Input: part model. Units: mm. Frame: model coordinates. Give positions to 0.01 mm unless a question says otherwise; leave off trailing zeros. Order: outer loops, then holes, each group sorted by start corner. A loop starts at its lowest first (then second) coordinate and runs counter-clockwise, first axis right, second up. Notation, with made-up numbers: (-26.5, 2) - (13.5, 2) arc R26 cw to (13.5, 21) - close; hole circle Ø1 at (19, 68). An arc over 180 degrees is marked (long way). Answer in a Markdown table with one row per item. Add a question column.
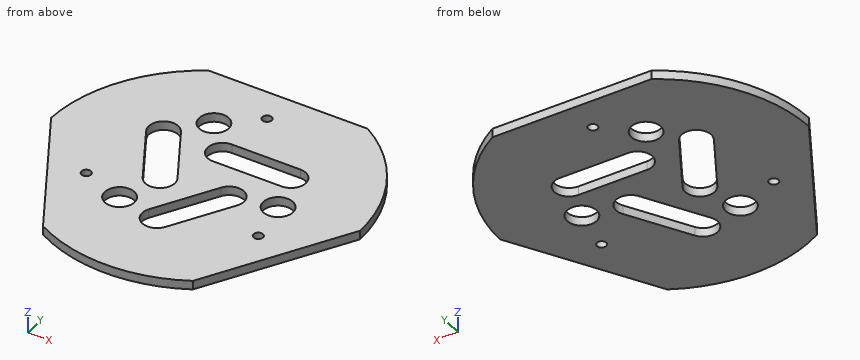
from build123d import *

# Parameters (mm, degrees)
SKETCH_1_R               = 1.6
SKETCH_1_R_2             = 5
EXTRUDE_1_DEPTH          = 1.5
CUT_EXTRUDE_1_DEPTH      = 75.301116494
PATTERN_CIRCULAR_1_COUNT = 3
SKETCH_3_R               = 5
CUT_EXTRUDE_3_DEPTH      = 75.301116494
PATTERN_CIRCULAR_3_COUNT = 3


with BuildPart() as part:
    # 草图1 → 凸台-拉伸1 (new, symmetric)
    with BuildSketch(Plane.XY):
        with BuildLine():
            Line((25.450325887, -45.918742494), (52.491960453, 0.918742494))
            ThreePointArc((52.491960453, 0.918742494), (45.466333699, 26.25), (27.041634566, 45))
            Line((27.041634566, 45), (-27.041634566, 45))
            ThreePointArc((-27.041634566, 45), (-45.466333699, 26.25), (-52.491960453, 0.918742494))
            Line((-52.491960453, 0.918742494), (-25.450325887, -45.918742494))
            ThreePointArc((-25.450325887, -45.918742494), (0, -52.5), (25.450325887, -45.918742494))
        make_face()
        with Locations((0, 33.75)):
            Circle(SKETCH_1_R, mode=Mode.SUBTRACT)
        with Locations((29.228357378, -16.875)):
            Circle(SKETCH_1_R, mode=Mode.SUBTRACT)
        with Locations((-29.228357378, -16.875)):
            Circle(SKETCH_1_R, mode=Mode.SUBTRACT)
        with Locations((0, -25)):
            Circle(SKETCH_1_R_2, mode=Mode.SUBTRACT)
        with Locations((-21.650635095, 12.5)):
            Circle(SKETCH_1_R_2, mode=Mode.SUBTRACT)
        with Locations((21.650635095, 12.5)):
            Circle(SKETCH_1_R_2, mode=Mode.SUBTRACT)
    extrude(amount=EXTRUDE_1_DEPTH, both=True)

    # 草图2 → 切除-拉伸1 (cut, through all)
    with BuildSketch(Plane.XY.offset(1.5)):
        with BuildLine():
            Line((-17.320508076, 15), (-5.669872981, -5.179491924))
            ThreePointArc((-5.669872981, -5.179491924), (-7.5, -12.009618943), (-14.330127019, -10.179491924))
            Line((-14.330127019, -10.179491924), (-25.980762114, 10))
            ThreePointArc((-25.980762114, 10), (-24.150635095, 16.830127019), (-17.320508076, 15))
        make_face()
    cut_extrude_1 = extrude(amount=-CUT_EXTRUDE_1_DEPTH, mode=Mode.SUBTRACT)

    # 阵列(圆周)1: 切除-拉伸1 ×3 about axis
    pattern_circular_1_axis = Axis((0, 0, 0), (0, 0, 1))
    for i in range(1, PATTERN_CIRCULAR_1_COUNT):
        add(cut_extrude_1.rotate(pattern_circular_1_axis, i * 360 / PATTERN_CIRCULAR_1_COUNT), mode=Mode.SUBTRACT)

    # 草图3 → 切除-拉伸3 (cut, through all)
    with BuildSketch(Plane.XY.offset(1.5)):
        with Locations((-11.650635095, 23.680339887)):
            Circle(SKETCH_3_R)
    cut_extrude_3 = extrude(amount=-CUT_EXTRUDE_3_DEPTH, mode=Mode.SUBTRACT)

    # 阵列(圆周)3: 切除-拉伸3 ×3 about axis
    pattern_circular_3_axis = Axis((0, 0, 0), (0, 0, 1))
    for i in range(1, PATTERN_CIRCULAR_3_COUNT):
        add(cut_extrude_3.rotate(pattern_circular_3_axis, i * 360 / PATTERN_CIRCULAR_3_COUNT), mode=Mode.SUBTRACT)


solid = part.part
Q1. Section C-C, the plane y = -25. Return loops of the section in (x, z), then the cut area to 3 significant figures.
Q2. Section A-A, the plane x = 0. Return loops of the section in (y, z).
Q3. Section B-B, the plane z = 0.9. State how many separate pieces and enclosed holes the cut face has, then the cut area to 3 significant figures.
Q4. Line query: probe 1 along X at (y, z) = (-10.5, -0.7); probe 2 along X at (y, z) = (-23.5, 1.2); probe 3 along Y at (x, z) = (23.5, 1.2). Output: solid intervals per line, ascending.
Q5. Section D-D, the plane y = 22.5. Return loops of the section in (x, z), then the cut area to 3 significant figures.
Q6. Contact query for flat-ended pins moving along their axis: P1, Ø16, axis at x = -11.65, y = 23.68, coming from the -Z side; P2, Ø1.5, axis at x = 10, z = 0, coming from the -Y side. Output: stop coordinate, or through.
Computed:
| question | item | result |
|---|---|---|
| 1 | outline | (-37.53, -1.5) - (-18.63, -1.5) - (-18.63, 1.5) - (-37.53, 1.5) - close; (-10.74, -1.5) - (-5, -1.5) - (-5, 1.5) - (-10.74, 1.5) - close; (5.77, -1.5) - (37.53, -1.5) - (37.53, 1.5) - (5.77, 1.5) - close |
| 1 | area | 169 mm^2 |
| 2 | outline | (-52.5, -1.5) - (-30, -1.5) - (-30, 1.5) - (-52.5, 1.5) - close; (-15, -1.5) - (7.5, -1.5) - (7.5, 1.5) - (-15, 1.5) - close; (17.5, -1.5) - (32.15, -1.5) - (32.15, 1.5) - (17.5, 1.5) - close; (35.35, -1.5) - (45, -1.5) - (45, 1.5) - (35.35, 1.5) - close |
| 3 | separate pieces | 1 |
| 3 | enclosed holes | 9 |
| 3 | area | 6,640 mm^2 |
| 4 | probe 1 | x = -45.9 to -14.13, -5.87 to 2.6, 14.15 to 45.9 |
| 4 | probe 2 | x = -38.39 to -19.43, -9.94 to -4.77, 6.64 to 38.39 |
| 4 | probe 3 | y = -46.95 to -5.87, 2.37 to 7.85, 17.15 to 45 |
| 5 | outline | (-47.43, -1.5) - (-16.51, -1.5) - (-16.51, 1.5) - (-47.43, 1.5) - close; (-6.79, -1.5) - (47.43, -1.5) - (47.43, 1.5) - (-6.79, 1.5) - close |
| 5 | area | 255 mm^2 |
| 6 | P1 | stops at z = -1.5 |
| 6 | P2 | stops at y = -51.68 |
